For this review, take the finished solid that the model builds, in its own axes (mm). Face numbers are marked on the shaded views. Coordinates: 2 decimals unless noted, no trailing zeros. Loops run counter-clockwise (first coordinate to the right, second up) from the corner with the lowest first, then second, coordinate; pieces in that order, holes last. Notation, with made-up numbers: (-20.5, -13.5) -> (16.5, -13.5) arc R13 ccw to (16.5, 3.5) -> close; hole circle Ø8 at (72.25, 18.5). An arc over 180 degrees is marked (long way). Answer in a Markdown table with one row per item.
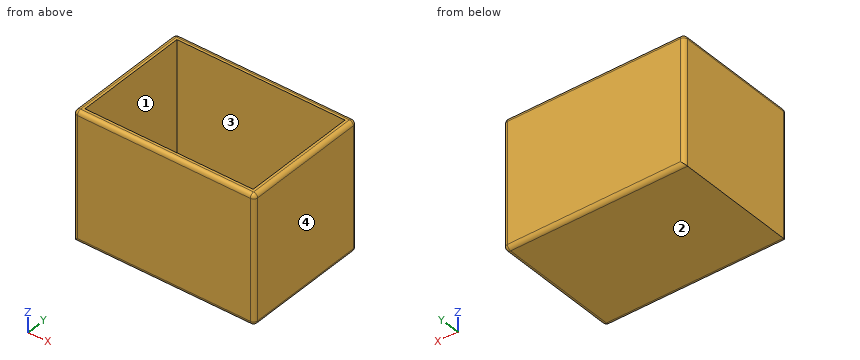
from build123d import *

# Parameters (mm, degrees)
F0_W     = 113
F0_H     = 80
F1_DEPTH = 80
F2_T     = -4
F3_R     = 2.5


with BuildPart() as f1:
    # F0 (on Front) → F1 (new body)
    with BuildSketch(Plane.XZ):
        with Locations((-56.5, 40)):
            Rectangle(F0_W, F0_H)
    extrude(amount=F1_DEPTH)

    # F2
    f2_openings = [f1.faces().sort_by_distance(p)[0] for p in [
        (-56.5, -40, 80),
    ]]
    offset(amount=F2_T, openings=f2_openings)

    # F3
    f3_edges = [f1.edges().sort_by_distance(p)[0] for p in [
        (0, -80, 40),
        (0, 0, 40),
        (0, -40, 80),
        (-56.5, -80, 80),
        (-56.5, 0, 80),
        (-56.5, -80, 0),
        (0, -40, 0),
        (-56.5, 0, 0),
        (-113, -80, 40),
        (-113, 0, 40),
        (-113, -40, 80),
    ]]
    fillet(f3_edges, radius=F3_R)


solid = f1.part
Item 1: Take a section at B-B, the plane x = -100. State the section outline as (y, z) points, and give its area (3 significant figures).
Worked answers:
| item | result |
|---|---|
| outline | (-80, 2.5) arc R2.5 ccw to (-77.5, 0) -> (-2.5, 0) arc R2.5 ccw to (0, 2.5) -> (0, 77.5) arc R2.5 ccw to (-2.5, 80) -> (-4, 80) -> (-4, 4) -> (-76, 4) -> (-76, 80) -> (-77.5, 80) arc R2.5 ccw to (-80, 77.5) -> close |
| area | 923 mm² |
Item 2: Take a section at C-C, the plane y = -38. State the section outline as (x, z) points, and give its area (3 significant figures).
Worked answers:
| item | result |
|---|---|
| outline | (-113, 0) -> (-2.5, 0) arc R2.5 ccw to (0, 2.5) -> (0, 77.5) arc R2.5 ccw to (-2.5, 80) -> (-4, 80) -> (-4, 4) -> (-109, 4) -> (-109, 80) -> (-110.5, 80) arc R2.5 ccw to (-113, 77.5) -> close |
| area | 1,060 mm² |
Item 3: Take a section at A-A, the plane z = 25. State the section outline as (x, y) points, and give its area (3 significant figures).
Worked answers:
| item | result |
|---|---|
| outline | (-113, -77.5) arc R2.5 ccw to (-110.5, -80) -> (-2.5, -80) arc R2.5 ccw to (0, -77.5) -> (0, -2.5) arc R2.5 ccw to (-2.5, 0) -> (-110.5, 0) arc R2.5 ccw to (-113, -2.5) -> close; hole (-109, -76) -> (-4, -76) -> (-4, -4) -> (-109, -4) -> close |
| area | 1,470 mm² |
Item 4: Insertion check: pin 1 (21.5 mm diameter, centred on x = -68, y = -53.5, fed in from +Z). The pin has a flat end and moves straight along its axis. Give the tip position at first contact, or say it passes through.
Worked answers:
| item | result |
|---|---|
| pin 1 | z = 4 |
Item 5: For L1, parallel to X at y = -50, z = 30; L2, parallel to Y at x = -102.5, z = 9; L3, parallel to Z at x = -38.5, y = -35.5, list the stretches that pass through material, from the lowest coordinate up.
Worked answers:
| item | result |
|---|---|
| L1 | -113 to -109, -4 to 0 |
| L2 | -80 to -76, -4 to 0 |
| L3 | 0 to 4 |
Item 6: The part is to be moulded in two halves that separate along X. For the marked faces 1, 2, 3 and 4, say which applies: +X half, -X half, draft (parallel to the pull), parting line (faces both ways), or undercut.
Worked answers:
| item | result |
|---|---|
| face 1 | undercut |
| face 2 | draft |
| face 3 | undercut |
| face 4 | +X half |
